```python
from build123d import *

# Parameters (mm, degrees)
F1_DEPTH = 127
F3_DEPTH = 0.4064


# Not quite as in the source:
# - the dataset's text gives a spline's control points without its knots; the knots are read off the source's solid


with BuildPart() as f1:
    # F0 (on Right) → F1 (new body, symmetric)
    with BuildSketch(Plane.YZ):
        Polygon((-139.7, 0), (0, 0), (0, 88.9), (-139.2936, 88.9), (-139.2936, 89.154), (-40.6298144724, 187.8177855276), (-40.9171826682, 188.1051537235), (-139.7, 89.3223363917), align=None)
    extrude(amount=F1_DEPTH, both=True)

    # F2 (on face) → F3 (cut, through all)
    with BuildSketch(Plane(origin=(0, -114.5111681959, 114.5111681959), x_dir=(1, 0, 0), z_dir=(0, -0.7071067812, 0.7071067812))):
        with BuildLine():
            add(Edge.make_bspline(
                [(-21.0882612312, 45.5766371575), (-17.1946190312, 49.4705841575), (-14.9277452312, 54.9434713575), (-14.9277452312, 60.4501405575), (-14.9277452312, 65.9570891575), (-17.1946190312, 71.4299763575), (-21.0882612312, 75.3236185575), (-24.9822590312, 79.2176163575), (-30.4551462312, 81.4845155575), (-35.9621202312, 81.4845155575)],
                knots=[5, 5, 5, 5, 6, 6, 6, 7, 7, 7, 8, 8, 8, 8], degree=3))
            add(Edge.make_bspline(
                [(-35.9621202312, 81.4845155575), (-41.4687640312, 81.4845155575), (-46.9416512312, 79.2176163575), (-50.8352934312, 75.3236185575)],
                knots=[0, 0, 0, 0, 1, 1, 1, 1], degree=3))
            add(Edge.make_bspline(
                [(-50.8352934312, 75.3236185575), (-54.7292912312, 71.4299763575), (-56.9964952312, 65.9570891575), (-56.9964952312, 60.4501405575), (-56.9964952312, 54.9434713575), (-54.7292912312, 49.4705841575), (-50.8352934312, 45.5766371575)],
                knots=[1, 1, 1, 1, 2, 2, 2, 3, 3, 3, 3], degree=3))
            add(Edge.make_bspline(
                [(-50.8352934312, 45.5766371575), (-46.9416512312, 41.6829441575), (-41.4687640312, 39.4157655575), (-35.9621202312, 39.4157655575), (-30.4551462312, 39.4157655575), (-24.9822590312, 41.6829441575), (-21.0882612312, 45.5766371575)],
                knots=[3, 3, 3, 3, 4, 4, 4, 5, 5, 5, 5], degree=3))
        make_face()
        with BuildLine():
            add(Edge.make_bspline(
                [(48.7617387688, 45.5766371575), (52.6553809688, 49.4705841575), (54.9222547688, 54.9434713575), (54.9222547688, 60.4501405575), (54.9222547688, 65.9570891575), (52.6553809688, 71.4299763575), (48.7617387688, 75.3236185575), (44.8677409688, 79.2176163575), (39.3948537688, 81.4845155575), (33.8878797688, 81.4845155575)],
                knots=[5, 5, 5, 5, 6, 6, 6, 7, 7, 7, 8, 8, 8, 8], degree=3))
            add(Edge.make_bspline(
                [(33.8878797688, 81.4845155575), (28.3812359688, 81.4845155575), (22.9083487688, 79.2176163575), (19.0147065688, 75.3236185575)],
                knots=[0, 0, 0, 0, 1, 1, 1, 1], degree=3))
            add(Edge.make_bspline(
                [(19.0147065688, 75.3236185575), (15.1207087688, 71.4299763575), (12.8535047688, 65.9570891575), (12.8535047688, 60.4501405575), (12.8535047688, 54.9434713575), (15.1207087688, 49.4705841575), (19.0147065688, 45.5766371575)],
                knots=[1, 1, 1, 1, 2, 2, 2, 3, 3, 3, 3], degree=3))
            add(Edge.make_bspline(
                [(19.0147065688, 45.5766371575), (22.9083487688, 41.6829441575), (28.3812359688, 39.4157655575), (33.8878797688, 39.4157655575), (39.3948537688, 39.4157655575), (44.8677409688, 41.6829441575), (48.7617387688, 45.5766371575)],
                knots=[3, 3, 3, 3, 4, 4, 4, 5, 5, 5, 5], degree=3))
        make_face()
        with BuildLine():
            add(Edge.make_bspline(
                [(105.9117387688, 45.5766371575), (109.8053809688, 49.4705841575), (112.0722547688, 54.9434713575), (112.0722547688, 60.4501405575), (112.0722547688, 65.9570891575), (109.8053809688, 71.4299763575), (105.9117387688, 75.3236185575), (102.0177409688, 79.2176163575), (96.5448537688, 81.4845155575), (91.0378797688, 81.4845155575)],
                knots=[5, 5, 5, 5, 6, 6, 6, 7, 7, 7, 8, 8, 8, 8], degree=3))
            add(Edge.make_bspline(
                [(91.0378797688, 81.4845155575), (85.5312359688, 81.4845155575), (80.0583487688, 79.2176163575), (76.1647065688, 75.3236185575)],
                knots=[0, 0, 0, 0, 1, 1, 1, 1], degree=3))
            add(Edge.make_bspline(
                [(76.1647065688, 75.3236185575), (72.2707087688, 71.4299763575), (70.0035047688, 65.9570891575), (70.0035047688, 60.4501405575), (70.0035047688, 54.9434713575), (72.2707087688, 49.4705841575), (76.1647065688, 45.5766371575)],
                knots=[1, 1, 1, 1, 2, 2, 2, 3, 3, 3, 3], degree=3))
            add(Edge.make_bspline(
                [(76.1647065688, 45.5766371575), (80.0583487688, 41.6829441575), (85.5312359688, 39.4157655575), (91.0378797688, 39.4157655575), (96.5448537688, 39.4157655575), (102.0177409688, 41.6829441575), (105.9117387688, 45.5766371575)],
                knots=[3, 3, 3, 3, 4, 4, 4, 5, 5, 5, 5], degree=3))
        make_face()
        with BuildLine():
            add(Edge.make_bspline(
                [(-78.2382612312, 45.5766371575), (-74.3446190312, 49.4705841575), (-72.0777452312, 54.9434713575), (-72.0777452312, 60.4501405575), (-72.0777452312, 65.9570891575), (-74.3446190312, 71.4299763575), (-78.2382612312, 75.3236185575), (-82.1322590312, 79.2176163575), (-87.6051462312, 81.4845155575), (-93.1121202312, 81.4845155575)],
                knots=[5, 5, 5, 5, 6, 6, 6, 7, 7, 7, 8, 8, 8, 8], degree=3))
            add(Edge.make_bspline(
                [(-93.1121202312, 81.4845155575), (-98.6187640312, 81.4845155575), (-104.0916512312, 79.2176163575), (-107.9855982312, 75.3236185575)],
                knots=[0, 0, 0, 0, 1, 1, 1, 1], degree=3))
            add(Edge.make_bspline(
                [(-107.9855982312, 75.3236185575), (-111.8792912312, 71.4299763575), (-114.1464952312, 65.9570891575), (-114.1464952312, 60.4501405575), (-114.1464952312, 54.9434713575), (-111.8792912312, 49.4705841575), (-107.9855982312, 45.5766371575)],
                knots=[1, 1, 1, 1, 2, 2, 2, 3, 3, 3, 3], degree=3))
            add(Edge.make_bspline(
                [(-107.9855982312, 45.5766371575), (-104.0916512312, 41.6829441575), (-98.6187640312, 39.4157655575), (-93.1121202312, 39.4157655575), (-87.6051462312, 39.4157655575), (-82.1322590312, 41.6829441575), (-78.2382612312, 45.5766371575)],
                knots=[3, 3, 3, 3, 4, 4, 4, 5, 5, 5, 5], degree=3))
        make_face()
    extrude(amount=-F3_DEPTH, mode=Mode.SUBTRACT)


solid = f1.part
```
Model file for the job. Use its own axes, mm. A direction names the side the tool comes from. Give positions to 0.01 mm unless a question says otherwise; leave off trailing zeros. Write each loop counter-clockwise with the first axis right and the second up, starting at its lowest first coordinate (ties: lowest second). Pieces come first, ordered by that corner, then holes. Notation, with made-up numbers: (-38.75, 78.5) -> (-18.75, 78.5) arc R21 cw to (-18.75, 83.5) -> close; hole circle Ø11 at (-32.5, 53). An arc over 180 degrees is marked (long way). Use CSV: the item, a comma, the result in double quotes. Start each with the question number.
1) Pin check, flat tip, straight feed: P1, Ø12, axis at x = -68.5, y = -32.5, coming from the +Z side. Stop position of the tip, or through.
2) Cut at A-A on x = 59.5. List the corners of the cut face in (y, z).
3) Cut at B-B on y = -105. List the corners of the cut face in (x, z).
4) Drill centre lines: L1, parallel to Z at x = -18, y = -31; L2, parallel to Z at x = -85, y = -54.5; L3, parallel to Z at x = 98, y = -56. Where is each one in solid material? Low to high.
5) Tool access for faces 1 (the flat face through (1.778, -89.617, 139.405)), 2 (the flat face through (1.78, -90.65, 137.8)): list every direction of +Z, -Z, +X, -X, +Y, -Y with a clear straight run to the whole face (end or side of a thin tool).
6) Cut at C-C on z = 153. Count the separate pieces of the cut face and the enclosed holes in it, plus the area to 3 significant figures.
Final values:
1,P1,"stops at z = 88.9"
2,outline,"(-139.7, 0) -> (0, 0) -> (0, 88.9) -> (-139.29, 88.9) -> (-139.29, 89.15) -> (-40.63, 187.82) -> (-40.92, 188.11) -> (-139.7, 89.32) -> close"
3,outline,"(-127, 0) -> (127, 0) -> (127, 88.9) -> (-127, 88.9) -> close; (-127, 123.45) -> (127, 123.45) -> (127, 124.02) -> (-127, 124.02) -> close"
4,L1,"z = 0 to 88.9"
4,L2,"z = 0 to 88.9, 173.95 to 174.52"
4,L3,"z = 0 to 88.9, 172.45 to 173.02"
5,face 1,"+Z, +X, -X, -Y"
5,face 2,"+X, -X, +Y"
6,separate pieces,"5"
6,enclosed holes,"0"
6,area,"53.1 mm2"
